from build123d import *

# Parameters (mm, degrees)
F1_DEPTH = 25.4
F0_W     = 4.9641267397
F0_H     = 20.5680120253
F2_DEPTH = 25.4
F4_DEPTH = 1.778


with BuildPart() as f1:
    # F0 (on Front) → F1 (new body)
    with BuildSketch(Plane.XZ):
        with BuildLine():
            add(Edge.make_bspline(
                [(-2.5424052642, 13.4505262055), (1.1521358093, 13.6647690598), (4.9162748075, 13.6731126703), (8.3490842731, 13.4505262055)],
                knots=[0.4880703365, 0.4880703365, 0.4880703365, 0.4880703365, 0.5400106865, 0.5400106865, 0.5400106865, 0.5400106865], degree=3))
            Line((-2.5424052642, 13.4505262055), (8.3490842731, 13.4505262055))
        make_face()
    extrude(amount=F1_DEPTH)

    # F0 (on Front) → F2 (join)
    with BuildSketch(Plane.XZ):
        with BuildLine():
            add(Edge.make_bspline(
                [(-20.8785217255, -55.6273907423), (-21.8121267596, -33.4650030089), (-23.1454067557, -1.8149292086), (-25.1589760047, 10.3212946622), (-10.0779831552, 13.0135453506), (-2.5424052642, 13.4505262055)],
                knots=[0, 0, 0, 0, 0.2675796431, 0.3821301005, 0.4880703365, 0.4880703365, 0.4880703365, 0.4880703365], degree=3))
            Line((-20.8785217255, -55.6273907423), (19.4184854627, -55.6273907423))
            add(Edge.make_bspline(
                [(8.3490842731, 13.4505262055), (12.9609733748, 13.1514871526), (24.0264096091, 11.1780304821), (21.9504869715, -2.2184048812), (20.4485582955, -33.8994631834), (19.4184854627, -55.6273907423)],
                knots=[0.5400106865, 0.5400106865, 0.5400106865, 0.5400106865, 0.6097911787, 0.732381762, 1, 1, 1, 1], degree=3))
            Line((8.3490842731, 13.4505262055), (-2.5424052642, 13.4505262055))
        make_face()
        with BuildLine():
            Line((-7.7423275904, 13.4505262055), (-2.5424052642, 13.4505262055))
            add(Edge.make_bspline(
                [(-2.5424052642, 13.4505262055), (1.1521358093, 13.6647690598), (4.9162748075, 13.6731126703), (8.3490842731, 13.4505262055)],
                knots=[0.4880703365, 0.4880703365, 0.4880703365, 0.4880703365, 0.5400106865, 0.5400106865, 0.5400106865, 0.5400106865], degree=3))
            Line((8.3490842731, 13.4505262055), (8.3490842731, 21.6907939184))
            Line((8.3490842731, 21.6907939184), (2.4820633698, 21.6907939184))
            Line((2.4820633698, 21.6907939184), (-2.4820633698, 21.6907939184))
            Line((-2.4820633698, 21.6907939184), (-7.7423275904, 21.6907939184))
            Line((-7.7423275904, 21.6907939184), (-7.7423275904, 13.4505262055))
        make_face()
        with BuildLine():
            add(Edge.make_bspline(
                [(-2.5424052642, 13.4505262055), (1.1521358093, 13.6647690598), (4.9162748075, 13.6731126703), (8.3490842731, 13.4505262055)],
                knots=[0.4880703365, 0.4880703365, 0.4880703365, 0.4880703365, 0.5400106865, 0.5400106865, 0.5400106865, 0.5400106865], degree=3))
            Line((-2.5424052642, 13.4505262055), (8.3490842731, 13.4505262055))
        make_face()
        with Locations((0, 31.974799931)):
            Rectangle(F0_W, F0_H)
    extrude(amount=F2_DEPTH)

    # F3 (on face) → F4 (join)
    with BuildSketch(Plane.XY.offset(42.2588059437)):
        with BuildLine():
            add(Edge.make_bspline(
                [(1.8980501918, -12.7), (1.8980501918, -5.0506086184), (-24.8206210672, -8.8753043092), (-51.5392923262, -12.7), (-24.8206210672, -16.5246956908), (1.8980501918, -20.3493913816), (1.8980501918, -12.7)],
                knots=[0, 0, 0, 2.0943951024, 2.0943951024, 4.1887902048, 4.1887902048, 6.2831853072, 6.2831853072, 6.2831853072], degree=2, weights=[1, 0.5, 1, 0.5, 1, 0.5, 1]))
        make_face()
    extrude(amount=-F4_DEPTH)


solid = f1.part
The listing builds one solid part. Answer for the finished solid, in the listing's coordinates (mm). A direction names the side the tool comes from. Round coordinates to 2 decimals unless told otherwise and drop trailing zeros. Write each question's results on one line, items separated by ' | '. Start each with the question number.
Item 1: Straight lines are drawn through the part: L1, parallel to X at y = -13, z = 34; L2, parallel to X at y = -17.75, z = 18; L3, parallel to Z at x = 3, y = -23.75. For each, find the intervals that lie inside material, in ascending order. Write a range as [from, to].
Item 2: Flat-ended cylindrical pins translate along their axes: pin 1 Ø10 at (y, z) = (-20.5, -41.5) entering from +X; pin 2 Ø1.8 at (x, y) = (7, -12.5) entering from +Z; pin 3 Ø8 at (y, z) = (-20, 11.5) entering from +X; pin 4 Ø2 at (x, z) = (-23, -40) entering from -Y. Find the tip coordinate at first contact, or state that the pin passes through.
Item 3: For faces 1 (the face through (8.349, -13, 18)), 2 (the face through (-7.742, -13, 18)), 3 (the face through (-1, -13, -55.627)), determine the directions among +Z, -Z, +X, -X, +Y, -Y from which every point of the face is accessible in a straight line to the end or side of a thin tool.
Check sheet entries:
1) L1: [-2.48, 2.48] | L2: [-7.74, 8.35] | L3: [-55.63, 21.69]
2) pin 1: x = 20.34 | pin 2: z = 21.69 | pin 3: x = 22.71 | pin 4: through
3) face 1: +Z, +X, +Y, -Y | face 2: -X, +Y, -Y | face 3: -Z, +X, -X, +Y, -Y
